```python
from build123d import *

# Parameters (mm, degrees)
SKETCH1_R                = 12.7
BOSS_EXTRUDE1_DEPTH      = 7.9375
SKETCH3_R                = 7.62
CUT_EXTRUDE2_DEPTH       = 20.636290542
SKETCH4_R                = 11.176
CUT_EXTRUDE3_DEPTH       = 7.112
BOSS_EXTRUDE2_START      = -3.175
BOSS_EXTRUDE2_DEPTH      = 3.175
SKETCH6_R                = 1.9
CUT_EXTRUDE4_DEPTH       = 26.242747597
FILLET1_R                = 3.175
CIRPATTERN1_COUNT        = 2
FILLET1_OF_CIRPATTERN1_R = 3.175
FILLET2_R                = 1.5875


with BuildPart() as part:
    # Sketch1 → Boss-Extrude1 (new body)
    with BuildSketch(Plane(origin=(0, 0, 0), x_dir=(1, 0, 0), z_dir=(0, 1, 0))):
        with Locations(Location((0, 0, 0), (0, 0, 270))):
            Circle(SKETCH1_R)
    extrude(amount=BOSS_EXTRUDE1_DEPTH)

    # Sketch3 → Cut-Extrude2 (cut, through all)
    with BuildSketch(Plane(origin=(0, 7.9375, 0), x_dir=(1, 0, 0), z_dir=(0, 1, 0))):
        with Locations(Location((0, 0, 0), (0, 0, 270))):
            Circle(SKETCH3_R)
    extrude(amount=-CUT_EXTRUDE2_DEPTH, mode=Mode.SUBTRACT)

    # Sketch4 → Cut-Extrude3 (cut)
    with BuildSketch(Plane(origin=(0, 7.9375, 0), x_dir=(1, 0, 0), z_dir=(0, 1, 0))):
        with Locations(Location((0, 0, 0), (0, 0, 270))):
            Circle(SKETCH4_R)
    extrude(amount=-CUT_EXTRUDE3_DEPTH, mode=Mode.SUBTRACT)

    # Sketch5 → Boss-Extrude2 (add)
    with BuildSketch(Plane(origin=(0, 7.9375, 0), x_dir=(1, 0, 0), z_dir=(0, 1, 0)).offset(BOSS_EXTRUDE2_START)):
        with BuildLine():
            Line((-4.7625, 11.773215098), (-4.7625, 20.32))
            Line((-4.7625, 20.32), (4.7625, 20.32))
            Line((4.7625, 20.32), (4.7625, 11.773215098))
            ThreePointArc((4.7625, 11.773215098), (0, 12.7), (-4.7625, 11.773215098))
        make_face()
    boss_extrude2 = extrude(amount=BOSS_EXTRUDE2_DEPTH)

    # Sketch6 → Cut-Extrude4 (cut, symmetric)
    with BuildSketch(Plane(origin=(0, 7.9375, 0), x_dir=(1, 0, 0), z_dir=(0, 1, 0))):
        with Locations(Location((0, 16.51, 0), (0, 0, 270))):
            Circle(SKETCH6_R)
    cut_extrude4 = extrude(amount=CUT_EXTRUDE4_DEPTH, both=True, mode=Mode.SUBTRACT)

    # Fillet1
    fillet1_edges = [part.edges().sort_by_distance(p)[0] for p in [
        (-4.7625, 6.35, -20.32),
        (4.7625, 6.35, -20.32),
    ]]
    fillet(fillet1_edges, radius=FILLET1_R)

    # CirPattern1: Boss-Extrude2, Cut-Extrude4 ×2 about axis
    cirpattern1_axis = Axis((0, 0, 0), (0, 1, 0))
    add([boss_extrude2.rotate(cirpattern1_axis, i * 360 / CIRPATTERN1_COUNT) for i in range(1, CIRPATTERN1_COUNT)])
    add([cut_extrude4.rotate(cirpattern1_axis, i * 360 / CIRPATTERN1_COUNT) for i in range(1, CIRPATTERN1_COUNT)], mode=Mode.SUBTRACT)

    # Fillet1 of CirPattern1
    fillet1_of_cirpattern1_edges = [part.edges().sort_by_distance(p)[0] for p in [
        (4.7625, 6.35, 20.32),
        (-4.7625, 6.35, 20.32),
    ]]
    fillet(fillet1_of_cirpattern1_edges, radius=FILLET1_OF_CIRPATTERN1_R)

    # Fillet2
    fillet2_edges = [part.edges().sort_by_distance(p)[0] for p in [
        (0, 4.7625, -12.7),
        (4.7625, 6.35, -11.773215098),
        (-4.7625, 6.35, -11.773215098),
        (0, 0, -12.7),
        (-2.425919233, 4.7625, 12.466150804),
        (-4.7625, 6.35, 11.773215098),
        (4.7625, 6.35, 11.773215098),
    ]]
    fillet(fillet2_edges, radius=FILLET2_R)


solid = part.part
```
Geometry: final body of the model. Coordinates: model frame, mm. A direction names the side the tool comes from. Round coordinates to 2 decimals unless told otherwise and drop trailing zeros. Write each loop counter-clockwise with the first axis right and the second up, starting at its lowest first coordinate (ties: lowest second). Pieces come first, ordered by that corner, then holes.
Item 1: Set-up query: faces 1 (the face through (4.762, 6, 15)), 2 (the face through (-4.763, 6, 15)), 3 (the face through (4.762, 6, -15)), 4 (the face through (-10.91, 4.43, -2.42)). Return all of +Z, -Z, +X, -X, +Y, -Y with unobstructed straight access to the full face (end or side cutting, diameter ignored); none if empty.
Item 2: Material intervals for L1, parallel to X at y = 6.75, z = -16.51; L2, parallel to Z at x = 6.25, y = 6.5; L3, parallel to X at y = 6.75, z = 0, sorted ascending.
Item 3: Section query A-A (z = 16.51). Return loops of the section in (x, y), plus the area to 3 significant figures.
Item 4: Pin query (flat end, axial travel): P1, Ø2, axis at x = 1, z = 17.5, coming from the -Y side; P2, Ø2, axis at x = -5.5, z = -12, coming from the -Y side; P3, Ø10, axis at x = -9.5, z = -3.5, coming from the -Y side; P4, Ø1, axis at y = 6, z = 15, coming from the -X side. Return the tip coordinate at first contact, or that it passes through.
Item 5: Section query B-B (x = 0). Give the number of separate pieces and of enclosed holes in the cut face, plus the area to 3 significant figures.
Item 6: Section query D-D (y = 2.5). Return loops of the section in (x, z).
Item 7: Mould query, pull axis Z, two halves, no side actions, for faces 5 (the face through (3.857, 6.372, -19.365)), 6 (the face through (-0.08, 6.37, 18.41)), 7 (the face through (0.08, 6.37, -18.41)), 8 (the face through (-4.762, 6, -15)). Classes: +Z half, -Z half, draft (parallel to the pull), parting line (faces both ways), or undercut.
Completed:
1. face 1: +Z, +X, +Y, -Y
1. face 2: +Z, -X, +Y, -Y
1. face 3: -Z, +X, +Y, -Y
1. face 4: +Y
2. L1: x = -4.76 to -1.9, 1.9 to 4.76
2. L2: z = -11.06 to -9.27, 9.27 to 11.06
2. L3: x = -12.7 to -11.18, 11.18 to 12.7
3. outline: (-4.76, 4.76) - (-1.9, 4.76) - (-1.9, 7.94) - (-4.76, 7.94) - close; (1.9, 4.76) - (4.76, 4.76) - (4.76, 7.94) - (1.9, 7.94) - close
3. area: 18.2 mm2
4. P1: stops at y = 4.76
4. P2: stops at y = 0.43
4. P3: stops at y = 0
4. P4: stops at x = -4.76
5. separate pieces: 4
5. enclosed holes: 0
5. area: 54.3 mm2
6. outline: circle Ø25.4 at (0, 0); hole circle Ø22.35 at (0, 0)
7. face 5: -Z half
7. face 6: undercut
7. face 7: undercut
7. face 8: draft
